Could you check a few things on this model? Use its own coordinates, in mm. Face numbers are marked on the shaded views. A direction names the side the tool comes from. Round coordinates to 2 decimals unless told otherwise and drop trailing zeros. Write each loop counter-clockwise with the first axis right and the second up, starting at its lowest first coordinate (ties: lowest second). Pieces come first, ordered by that corner, then holes. Notation, with made-up numbers: M -29.5,-6.75 L -17.5,-6.75 A12 ccw -17.5,3.25 Z; hole C 51,71 d5. An arc over 180 degrees is marked long. One line per item, written item: value. Start each with the question number.
(1) I want a section at D-D on x = 6. Please give me the cut outline in (y, z).
(2) I want a section at A-A on z = 0. Please give me the cut outline in (x, y).
(3) Which directions (+Z, -Z, +X, -X, +Y, -Y) give clear straight access to the entire face, cutting with the end or side of a thin tool? Please do the marked faces 1, 2 and 3.
(4) If I drill on L1, parallel to Y at x = 2.25, z = -7.25; L2, parallel to X at y = 35.5, z = -0.5; L3, parallel to Y at x = 0.5, z = 4.5, over which ranges is the centre line in solid material (lowest first)?
(5) Thinking about a two-plate mould opening in Y: for the marked faces 4, 5 and 6, which applies, released by +Y, released by -Y, zero draft, split by the parting line, or undercut?
(6) I want a section at B-B on y = 47.5. Please give me the cut outline in (x, z).
(7) I want a section at C-C on y = 58. Please give me the cut outline in (x, z).
(8) I'm going to push flat-ended pins straight in: pin 1 Ø2 at (x, z) = (-4.5, 4) entering from +Y; pin 2 Ø5 at (y, z) = (19.5, 1.5) entering from -X; pin 3 Ø1.5 at (x, z) = (1, -2.5) entering from -Y; pin 4 Ø8 at (x, z) = (2, 5.5) entering from +Y. Where does each tip first touch, or does it pass through?
```python
from build123d import *

# Parameters (mm, degrees)
SKETCH1_R           = 3
BOSS_EXTRUDE1_DEPTH = 35
FILLET1_R           = 3
SKETCH2_R           = 5
BOSS_EXTRUDE2_DEPTH = 15
BOSS_EXTRUDE3_DEPTH = 6
SKETCH4_R           = 4
BOSS_EXTRUDE4_DEPTH = 20
FILLET2_R           = 3


with BuildPart() as part:
    # Sketch1 → Boss-Extrude1 (new body)
    with BuildSketch(Plane(origin=(0, 0, 0), x_dir=(1, 0, 0), z_dir=(0, 1, 0))):
        with Locations(Location((0, 0, 0), (0, 0, 270))):
            Circle(SKETCH1_R)
    extrude(amount=BOSS_EXTRUDE1_DEPTH)

    # Fillet1
    fillet1_edges = [part.edges().sort_by_distance(p)[0] for p in [
        (0, 0, -3),
    ]]
    fillet(fillet1_edges, radius=FILLET1_R)

    # Sketch2 → Boss-Extrude2 (add)
    with BuildSketch(Plane(origin=(0, 35, 0), x_dir=(1, 0, 0), z_dir=(0, 1, 0))):
        with Locations(Location((0, 0, 0), (0, 0, 270))):
            Circle(SKETCH2_R)
    extrude(amount=BOSS_EXTRUDE2_DEPTH)

    # Sketch3 → Boss-Extrude3 (add)
    with BuildSketch(Plane(origin=(0, 50, 0), x_dir=(1, 0, 0), z_dir=(0, 1, 0))):
        Polygon((7.75, -4.474464586), (7.75, 4.474464586), (0, 8.948929172), (-7.75, 4.474464586), (-7.75, -4.474464586), (0, -8.948929172), align=None)
    extrude(amount=BOSS_EXTRUDE3_DEPTH)

    # Sketch4 → Boss-Extrude4 (add)
    with BuildSketch(Plane(origin=(0, 56, 0), x_dir=(1, 0, 0), z_dir=(0, 1, 0))):
        with Locations(Location((0, 0, 0), (0, 0, 270))):
            Circle(SKETCH4_R)
    extrude(amount=BOSS_EXTRUDE4_DEPTH)

    # Fillet2
    # the kernel refuses this fillet: 3 mm, written as the material it adds along each edge
    with BuildSketch(Plane(origin=(0, 35, 0), x_dir=(0, 0, 1), z_dir=(-1, 0, 0))) as fillet2_piece_1:
        with BuildLine():
            CenterArc((6, -2.828427125), FILLET2_R, 109.471220634, 70.528779366)
            Line((3, -2.828427125), (2.94, -2.828427125))
            Line((2.94, -2.828427125), (2.94, 0))
            Line((2.94, 0), (3, 0.06))
            ThreePointArc((3, 0.06), (4, 0.06), (4.98, 0.056568542))
            Line((4.98, 0.056568542), (5, 0))
        make_face()
    revolve(axis=Axis((0, 35, 0), (0, 1, 0)))


solid = part.part
```
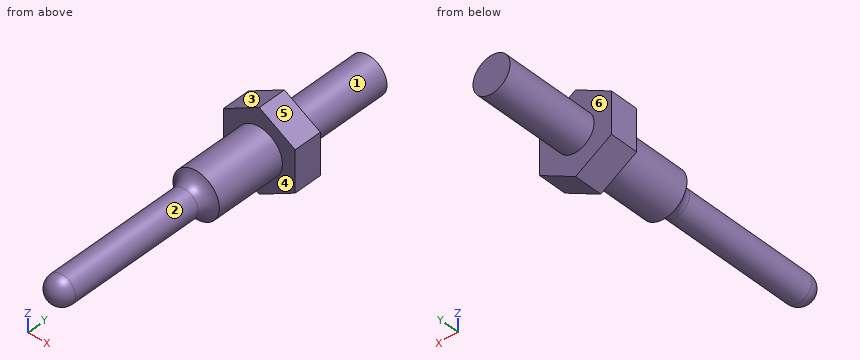
Found:
1. outline: M 50,-5.48 L 56,-5.48 L 56,5.48 L 50,5.48 Z
2. outline: M -7.75,50 L -5,50 L -5,35 A3 cw -3,32.17 L -3,3 A3 ccw 3,3 L 3,32.17 A3 cw 5,35 L 5,50 L 7.75,50 L 7.75,56 L 4,56 L 4,76 L -4,76 L -4,56 L -7.75,56 Z
3. face 1: +Y
3. face 2: -Y
3. face 3: +Z, -X, +Y, -Y
4. L1: y = 50 to 56
4. L2: x = -4.97 to 4.97
4. L3: y = 34.79 to 56
5. face 4: released by -Y
5. face 5: zero draft
5. face 6: released by +Y
6. outline: C 0,0 d10
7. outline: C 0,0 d8
8. pin 1: stops at y = 56
8. pin 2: stops at x = -3
8. pin 3: stops at y = 0.71
8. pin 4: stops at y = 76
